Could you check a few things on this model? Use its own coordinates, in mm. Coordinates: 2 decimals unless noted, no trailing zeros. Loops run counter-clockwise (first coordinate to the right, second up) from the corner with the lowest first, then second, coordinate; pieces in that order, holes last. Notation, with made-up numbers: (-21.5, -15.75) - (8.5, -15.75) arc R12 ccw to (8.5, -3.75) - close; hole circle Ø9 at (21.5, 64). An arc over 180 degrees is marked (long way). Use CSV: the item, a comma, the result in double quotes.
from build123d import *

# Parameters (mm, degrees)
F1_DEPTH = 8
F2_DEPTH = 3
F4_DEPTH = 11


with BuildPart() as f1:
    # F0 (on Front) → F1 (new body)
    with BuildSketch(Plane.XZ):
        with BuildLine():
            ThreePointArc((-30.0701617141, 46.3723698281), (-35.6321374629, 46.5684078352), (-41.1665091954, 47.1555489225))
            ThreePointArc((-41.1665091954, 47.1555489225), (-30.0701617141, -22.1997679505), (-18.9738142329, 47.1555489225))
            ThreePointArc((-18.9738142329, 47.1555489225), (-24.5081859654, 46.5684078352), (-30.0701617141, 46.3723698281))
        make_face()
        with BuildLine():
            ThreePointArc((-22.5701617141, 13.3655580288), (-35.373462573, 8.0622571699), (-30.0701617141, 20.8655580288))
            ThreePointArc((-30.0701617141, 20.8655580288), (-24.7668608552, 18.6688588877), (-22.5701617141, 13.3655580288))
        make_face(mode=Mode.SUBTRACT)
    extrude(amount=F1_DEPTH)

    # F0 (on Front) → F2 (join)
    with BuildSketch(Plane.XZ):
        with BuildLine():
            ThreePointArc((-30.0701617141, 56.2795021275), (-36.9667710759, 53.357462718), (-41.1665091954, 47.1555489225))
            ThreePointArc((-41.1665091954, 47.1555489225), (-35.6321374629, 46.5684078352), (-30.0701617141, 46.3723698281))
            Line((-30.0701617141, 46.3723698281), (-30.0701617141, 50.7215580288))
            ThreePointArc((-30.0701617141, 50.7215580288), (-32.0701617141, 52.7215580288), (-30.0701617141, 54.7215580288))
            Line((-30.0701617141, 54.7215580288), (-30.0701617141, 56.2795021275))
        make_face()
        with BuildLine():
            ThreePointArc((-30.0701617141, 46.3723698281), (-24.5081859654, 46.5684078352), (-18.9738142329, 47.1555489225))
            ThreePointArc((-18.9738142329, 47.1555489225), (-23.1735523524, 53.357462718), (-30.0701617141, 56.2795021275))
            Line((-30.0701617141, 56.2795021275), (-30.0701617141, 54.7215580288))
            ThreePointArc((-30.0701617141, 54.7215580288), (-28.6559481518, 54.1357715912), (-28.0701617141, 52.7215580288))
            ThreePointArc((-28.0701617141, 52.7215580288), (-28.6559481518, 51.3073444665), (-30.0701617141, 50.7215580288))
            Line((-30.0701617141, 50.7215580288), (-30.0701617141, 46.3723698281))
        make_face()
    extrude(amount=F2_DEPTH)


with BuildPart() as f4:
    # F0 (on Front) → F4 (new body)
    with BuildSketch(Plane.XZ):
        with BuildLine():
            ThreePointArc((-22.5701617141, 13.3655580288), (-24.7668608552, 18.6688588877), (-30.0701617141, 20.8655580288))
            ThreePointArc((-30.0701617141, 20.8655580288), (-35.373462573, 8.0622571699), (-22.5701617141, 13.3655580288))
        make_face()
        with BuildLine():
            ThreePointArc((-27.5701617141, 13.3655580288), (-31.8379286671, 11.5977910759), (-30.0701617141, 15.8655580288))
            ThreePointArc((-30.0701617141, 15.8655580288), (-28.3023947612, 15.1333249818), (-27.5701617141, 13.3655580288))
        make_face(mode=Mode.SUBTRACT)
    extrude(amount=F4_DEPTH)


solid = f4.part
(1) Suppose I cut it at B-B (y = -6.5). Write out the boundary of the cut face in (x, z).
Computed:
outline,"circle Ø15 at (-30.07, 13.37); hole circle Ø5 at (-30.07, 13.37)"
(2) Please list where these lines run through material, in increasing order: line 1 (X direction, y = -2, z = 13.25); line 2 (Z direction, x = -29.25, y = -3.25); line 3 (X direction, y = -1.75, z = 11.5).
Computed:
line 1,"x = -37.57 to -32.57, -27.57 to -22.57"
line 2,"z = 5.91 to 11, 15.73 to 20.82"
line 3,"x = -37.33 to -31.73, -28.41 to -22.81"
(3) Will these pins go through, and if not, where does the flat tip stop? pin 1 (1 mm diameter, centred on x = -35, y = -3.5, fed in from -Z); pin 2 (3 mm diameter, centred on y = -1.5, z = 17, fed in from +X); pin 3 (3 mm diameter, centred on x = -24.5, y = -3, fed in from -Z); pin 4 (3 mm diameter, centred on x = -30.07, z = 13.37, fed in from +Y) (3 decimals).
Computed:
pin 1,"stops at z = 7.31"
pin 2,"stops at x = -22.88"
pin 3,"stops at z = 7.07"
pin 4,"passes through"
(4) Suppose I cut it at A-A (x = -31). Write out the boundary of the cut face in (y, z), plus the area to 3 significant figures.
Computed:
outline,"(-11, 5.92) - (0, 5.92) - (0, 11.04) - (-11, 11.04) - close; (-11, 15.69) - (0, 15.69) - (0, 20.81) - (-11, 20.81) - close"
area,"113 mm²"
(5) Suppose I cut it at D-D (z = 9). Write out the boundary of the cut face in (x, y), plus the area to 3 significant figures.
Computed:
outline,"(-36.17, -11) - (-23.97, -11) - (-23.97, 0) - (-36.17, 0) - close"
area,"134 mm²"
(6) Suppose I cut it at C-C (x = -29). Write out the boundary of the cut face in (y, z).
Computed:
outline,"(-11, 5.94) - (0, 5.94) - (0, 11.11) - (-11, 11.11) - close; (-11, 15.62) - (0, 15.62) - (0, 20.79) - (-11, 20.79) - close"
